```python
from build123d import *

# Parameters (mm, degrees)
EXTRUDE_1_DEPTH    = 10
HOLE_WIZARD_M2_1_D = 2.4
CHAMFER_1_SIZE     = 1


with BuildPart() as part:
    # 草图3 → 凸台-拉伸1 (new body)
    with BuildSketch(Plane(origin=(3, 0, 0), x_dir=(0, 0, -1), z_dir=(1, 0, 0))):
        with BuildLine():
            Line((-7, -31), (0, -31))
            Line((0, -31), (0, -16))
            Line((0, -16), (-1.5, -16))
            ThreePointArc((-1.5, -16), (-2.914213562, -15.414213562), (-3.5, -14))
            Line((-3.5, -14), (-3.5, 0.5))
            Line((-3.5, 0.5), (-1, 0.5))
            Line((-1, 0.5), (-5.76701437, 4.5))
            Line((-5.76701437, 4.5), (-7, 4.5))
            Line((-7, 4.5), (-7, -31))
        make_face()
    extrude(amount=-EXTRUDE_1_DEPTH)

    # M2 间隙孔1 (through all)
    with Locations(Plane.XY.offset(7)):
        with Locations((-1, -26.5), (-3, -20.5)):
            Hole(HOLE_WIZARD_M2_1_D / 2)

    # 倒角1
    chamfer_1_edges = [part.edges().sort_by_distance(p)[0] for p in [
        (3, -13.25, 7),
        (-2, -31, 7),
        (-7, -13.25, 7),
    ]]
    chamfer(chamfer_1_edges, length=CHAMFER_1_SIZE)


solid = part.part
```
CAD build for the part. Positions are in the model's coordinates, mm. A direction names the side the tool comes from. Round coordinates to 2 decimals unless told otherwise and drop trailing zeros. Loops run counter-clockwise (first coordinate to the right, second up) from the corner with the lowest first, then second, coordinate; pieces in that order, holes last. Notation, with made-up numbers: (-9, 73.5) - (44, 73.5) arc R17 cw to (44, 93.5) - close; hole circle Ø7 at (75.5, 18). An arc over 180 degrees is marked (long way). Return JSON: item names as keys, results as strings. Group by question number.
Q1. Drill centre lines: line 1 along Y through (x, z) = (-3, 3); line 2 along Y through (x, z) = (-1, 3); line 3 along Z through (x, y) = (-0.75, -10). Where is each one in solid material? Low to high. Write a range as [from, to].
Q2. Two-plate mould, pull along Y, no slides. Class faces 1 (the face through (2.5, -13, 6.5)), 2 (the face through (-1.93, 2.47, 3.35)), 3 (the face through (-2, -16, 1)): +Y half, -Y half, draft (parallel to the pull), parting line (faces both ways), or undercut.
Q3. Band-saw the part on D-D on x = -5. Give the cut face in (y, z), plus the area to 3 significant figures.
Q4. Flat gauge pins, fed straight in: pin 1 Ø3 at (x, z) = (1.5, 1.5) entering from +Y; pin 2 Ø3 at (x, y) = (-2.5, -6) entering from -Z; pin 3 Ø0.8 at (x, z) = (-0.5, 0.5) entering from +Y. Where does each tip first touch, or does it go through?
Q5. Band-saw the part on C-C on z = 6.5. Give the cut face in (x, y).
Q6. Tool access for faces 4 (the face through (3, -17, 4)), 5 (the face through (-1.93, -15.43, 2.9)): list every direction of +Z, -Z, +X, -X, +Y, -Y with a clear straight run to the whole face (end or side of a thin tool).
Q7. Band-saw the part on B-B on y = -26.5. Give the cut face in (x, z).
Q8. Band-saw the part on A-A on x = -3. Give the cut face in (y, z).
Solutions:
{
 "1": {"line 1": "y = [-31, -21.7], [-19.3, -15.32], [0.5, 2.18]", "line 2": "y = [-31, -27.7], [-25.3, -15.32], [0.5, 2.18]", "line 3": "z = [3.5, 7]"},
 "2": {"face 1": "draft", "face 2": "+Y half", "face 3": "undercut"},
 "3": {"outline": "(-31, 0) - (-16, 0) - (-16, 1.5) arc R2 cw to (-14, 3.5) - (0.5, 3.5) - (0.5, 1) - (4.5, 5.77) - (4.5, 7) - (-30, 7) - (-31, 6) - close", "area": "178 mm^2"},
 "4": {"pin 1": "stops at y = 2.18", "pin 2": "stops at z = 3.5", "pin 3": "stops at y = -16"},
 "5": {"outline": "(-6.5, -30.5) - (2.5, -30.5) - (2.5, 4.5) - (-6.5, 4.5) - close; hole circle Ø2.4 at (-3, -20.5); hole circle Ø2.4 at (-1, -26.5)"},
 "6": {"face 4": "+Z, -Z, +X, +Y, -Y", "face 5": "-Z, +X, -X"},
 "7": {"outline": "(-7, 0) - (-2.2, 0) - (-2.2, 7) - (-6, 7) - (-7, 6) - close; (0.2, 0) - (3, 0) - (3, 6) - (2, 7) - (0.2, 7) - close"},
 "8": {"outline": "(-31, 0) - (-21.7, 0) - (-21.7, 7) - (-30, 7) - (-31, 6) - close; (-19.3, 0) - (-16, 0) - (-16, 1.5) arc R2 cw to (-14, 3.5) - (0.5, 3.5) - (0.5, 1) - (4.5, 5.77) - (4.5, 7) - (-19.3, 7) - close"}
}
